The drawing under review shows one solid part. Ordinate dimensions are in mm from its lowest x, y, z. A direction names the side the tool comes from. Coordinates: 2 decimals unless noted, no trailing zeros. Order: outer loops, then holes, each group sorted by start corner. A loop starts at its lowest first (then second) coordinate and runs counter-clockwise, first axis right, second up. Notation, with made-up numbers: (-18, 87.25) -> (34, 87.25) arc R13 cw to (34, 98.25) -> close; hole circle Ø8 at (42, 19). An arc over 180 degrees is marked (long way). Put each result on its own line as item: value.
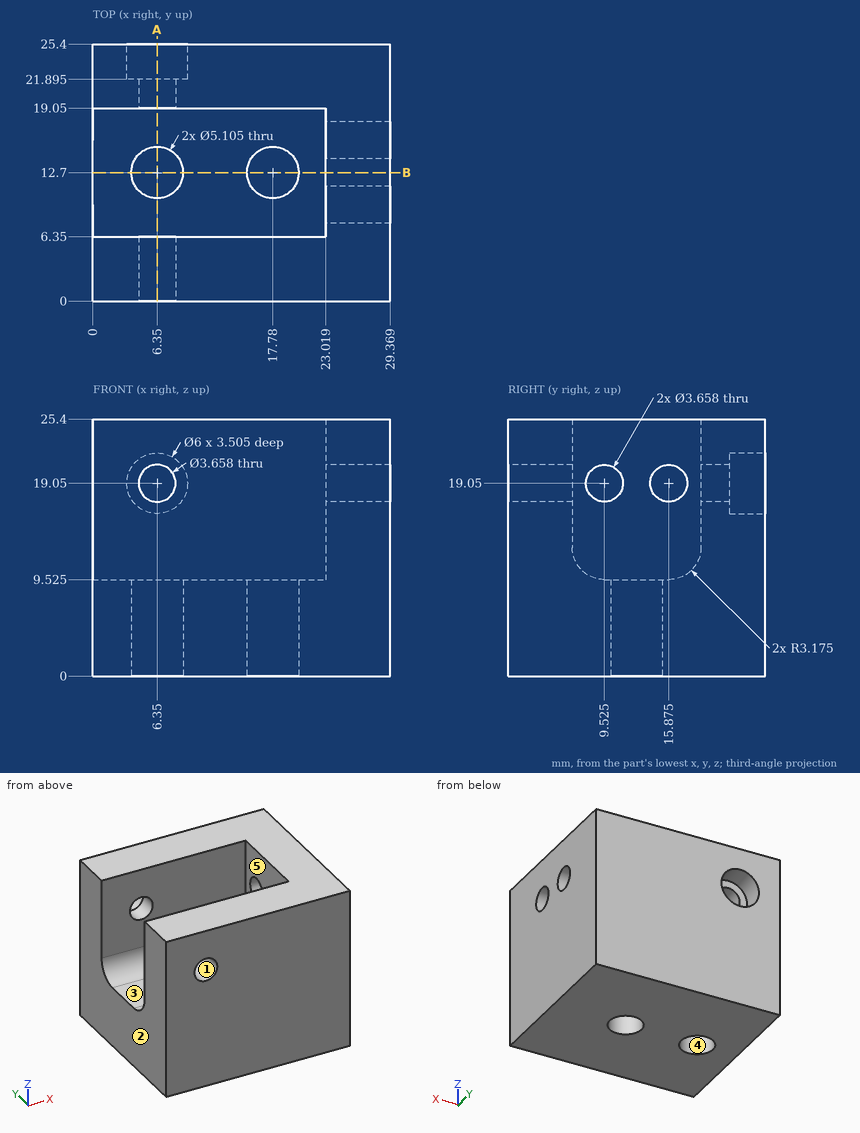
Item 1: Mouldability with a two-part tool opening along Z and no side actions: class the marked faces 1, 2 and 3 as +Z half, -Z half, draft (parallel to the pull), parting line (faces both ways), or undercut.
Answers below:
face 1: undercut
face 2: draft
face 3: +Z half
Item 2: For pin 1 Ø6 at (x, y) = (9, 8) entering from +Z; pin 2 Ø8 at (x, y) = (6.35, 12.7) entering from +Z; pin 3 Ø3 at (x, y) = (12.5, 15.5) entering from +Z; pin 4 Ø1.8 at (x, z) = (7.5, 18.5) entering from +Y (1 decimal), all flat-tipped, find the tip position at first contact; note any pin that passes through.
Answers below:
pin 1: z = 25.4
pin 2: z = 9.63
pin 3: z = 9.73
pin 4: y = 21.9
Item 3: For the marked faces 4 and 5, list the 3-axis set-ups (+Z, -Z, +X, -X, +Y, -Y) from which the entire face can be reached by the end or side of a thin tool; tool diameter is ignored.
Answers below:
face 4: +Z, -Z
face 5: +Z, -X
Item 4: Consider section A-A on x = 6.35. Count the separate pieces of the cut face and the enclosed holes in it.
Answers below:
separate pieces: 4
enclosed holes: 0
Item 5: Consider section B-B on y = 12.7. Write out the cut boundary in (x, z) (1 decimal), and give its area (3 significant figures).
Answers below:
outline: (0, 0) -> (3.8, 0) -> (3.8, 9.5) -> (0, 9.5) -> close; (8.9, 0) -> (15.2, 0) -> (15.2, 9.5) -> (8.9, 9.5) -> close; (20.3, 0) -> (29.4, 0) -> (29.4, 25.4) -> (23, 25.4) -> (23, 9.5) -> (20.3, 9.5) -> close
area: 283 mm^2
Item 6: For line 1 (Y direction, x = 6.35, z = 5.5); line 2 (X direction, y = 2.5, z = 19.05); line 3 (X direction, y = 23.1, z = 19.05), list the stretches that pass through material, from the lowest coordinate up. Write a range as from..to.
Answers below:
line 1: 0..10.15, 15.25..25.4
line 2: 0..4.52, 8.18..29.37
line 3: 0..3.35, 9.35..29.37
